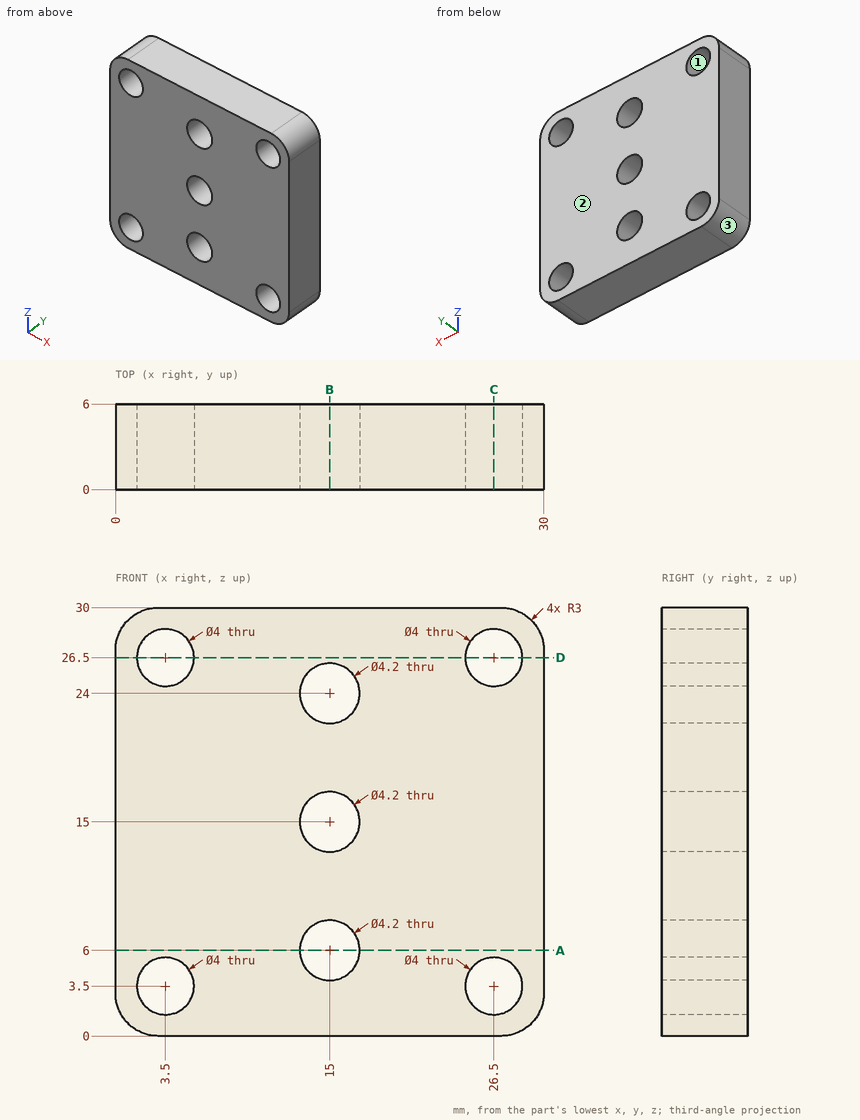
Geometry: see drawing. Coordinates: mm, zero at the bounding-box minimum. Round coordinates to 2 decimals unless told otherwise and drop trailing zeros. Order: outer loops, then holes, each group sorted by start corner. A loop starts at its lowest first (then second) coordinate and runs counter-clockwise, first axis right, second up. Notation, with made-up numbers: (-15.75, 60) - (39.25, 60) arc R31 cw to (39.25, 88) - close; hole circle Ø8 at (48, 33.25). An arc over 180 degrees is marked (long way). Use a Markdown table: item, result. Add a question column.
1. Section query D-D (z = 26.5). Return the cut outline in (x, y), then the cut area to 3 significant figures.
2. Section query C-C (x = 26.5). Return the cut outline in (y, z), then the cut area to 3 significant figures.
3. Section query A-A (z = 6). Return the cut outline in (x, y), then the cut area to 3 significant figures.
4. Mould query, pull axis Z, two halves, no side actions, for the marked faces 1, 2 and 3. Classes: +Z half, -Z half, draft (parallel to the pull), parting line (faces both ways), or undercut.
5. Section query B-B (x = 15). Return the cut outline in (y, z).
6. Line query: probe 1 along X at (y, z) = (4.45, 3.5); probe 2 along Z at (x, y) = (15, 3.6); probe 3 along X at (y, z) = (1.7, 15). Output: solid intervals per line, ascending.
Derived:
| question | item | result |
|---|---|---|
| 1 | outline | (0, 0) - (1.5, 0) - (1.5, 6) - (0, 6) - close; (5.5, 0) - (24.5, 0) - (24.5, 6) - (5.5, 6) - close; (28.5, 0) - (30, 0) - (30, 6) - (28.5, 6) - close |
| 1 | area | 132 mm2 |
| 2 | outline | (0, 0) - (6, 0) - (6, 1.5) - (0, 1.5) - close; (0, 5.5) - (6, 5.5) - (6, 24.5) - (0, 24.5) - close; (0, 28.5) - (6, 28.5) - (6, 30) - (0, 30) - close |
| 2 | area | 132 mm2 |
| 3 | outline | (0, 0) - (12.9, 0) - (12.9, 6) - (0, 6) - close; (17.1, 0) - (30, 0) - (30, 6) - (17.1, 6) - close |
| 3 | area | 155 mm2 |
| 4 | face 1 | undercut |
| 4 | face 2 | draft |
| 4 | face 3 | -Z half |
| 5 | outline | (0, 0) - (6, 0) - (6, 3.9) - (0, 3.9) - close; (0, 8.1) - (6, 8.1) - (6, 12.9) - (0, 12.9) - close; (0, 17.1) - (6, 17.1) - (6, 21.9) - (0, 21.9) - close; (0, 26.1) - (6, 26.1) - (6, 30) - (0, 30) - close |
| 6 | probe 1 | 0 to 1.5, 5.5 to 24.5, 28.5 to 30 |
| 6 | probe 2 | 0 to 3.9, 8.1 to 12.9, 17.1 to 21.9, 26.1 to 30 |
| 6 | probe 3 | 0 to 12.9, 17.1 to 30 |
